Autodesk Inventor part; units mm, degrees
ref_plane "YZ Plane" through (0, 0, 0) normal (1, 0, 0) x (0, 1, 0)
ref_plane "XZ Plane" through (0, 0, 0) normal (0, 1, 0) x (-1, 0, 0)
ref_plane "XY Plane" through (0, 0, 0) normal (0, 0, 1) x (1, 0, 0)
sketch "Skizze1" plane through (0, 0, 0) normal (0, 0, 1) x (1, 0, 0)
  line L0 (0, 0) -> (84, 0)
  line L1 (84, 0) -> (84, 48)
  line L2 (84, 48) -> (0, 48)
  line L3 (0, 48) -> (0, 0)
  dimension "d0" = 48
  dimension "d1" = 84
extrude "Extrusion1" add sketch "Skizze1" along normal blind 4
sketch "Skizze2" plane through (0, 0, 4) normal (0, 0, 1) x (1, 0, 0)
  line L0 (0, 48) -> (0, 0)
  line L1 (0, 0) -> (84, 0)
  line L2 (84, 0) -> (84, 48)
  point P0 (4, 12)
  point P1 (4, 42)
  point P2 (80, 42)
  point P3 (80, 12)
  dimension "d4" = 4
  dimension "d5" = 30
  dimension "d6" = 12
  dimension "d7" = 4
hole "Bohrung1" at (4, 12, 4) at (4, 42, 4) at (80, 42, 4) at (80, 12, 4) direction (0, 0, -1) diameter 4 depth 4
sketch "Skizze3" plane through (0, 0, 4) normal (0, 0, 1) x (1, 0, 0)
  line L0 (0, 0) -> (84, 0)
  line L1 (0, 48) -> (0, 0)
  point P0 (24, 4)
  point P1 (60, 4)
  dimension "d15" = 4
  dimension "d16" = 24
  dimension "d17" = 36
hole "Bohrung2" at (24, 4, 4) at (60, 4, 4) direction (0, 0, -1) diameter 4 depth 4
properties part number "1012"
The model under review builds one solid part; all positions refer to its coordinate system, in mm. Round coordinates to 2 decimals unless told otherwise and drop trailing zeros. Order: outer loops, then holes, each group sorted by start corner. A loop starts at its lowest first (then second) coordinate and runs counter-clockwise, first axis right, second up. Notation, with made-up numbers: (19, -12.5) -> (64, -12.5) arc R8 ccw to (64, -7.5) -> close; hole circle Ø1 at (-28, 1). An arc over 180 degrees is marked (long way). Use a Markdown table: item, result.
Q1. We need section C-C on z = 2.8. Write out the cut boundary in (x, y), then the cut area to 3 significant figures.
Values:
| item | result |
|---|---|
| outline | (0, 0) -> (84, 0) -> (84, 48) -> (0, 48) -> close; hole circle Ø4 at (4, 12); hole circle Ø4 at (4, 42); hole circle Ø4 at (24, 4); hole circle Ø4 at (60, 4); hole circle Ø4 at (80, 12); hole circle Ø4 at (80, 42) |
| area | 3,960 mm^2 |
Q2. Clearance check with a flat-ended pin moving along its axis: P1, Ø3.5, axis at x = 4, y = 42, coming from the -Z side. State where the tip first meets the part, or that it passes through.
Values:
| item | result |
|---|---|
| P1 | passes through |
Q3. We need section B-B on y = 12. Write out the cut boundary in (x, z).
Values:
| item | result |
|---|---|
| outline | (0, 0) -> (2, 0) -> (2, 4) -> (0, 4) -> close; (6, 0) -> (78, 0) -> (78, 4) -> (6, 4) -> close; (82, 0) -> (84, 0) -> (84, 4) -> (82, 4) -> close |
Q4. For line 1 (Y direction, x = 80, z = 1.8); line 2 (X direction, y = 42, z = 1.8); line 3 (X direction, y = 4, z = 0.9), list the stretches that pass through material, from the lowest coordinate up.
Values:
| item | result |
|---|---|
| line 1 | y = 0 to 10, 14 to 40, 44 to 48 |
| line 2 | x = 0 to 2, 6 to 78, 82 to 84 |
| line 3 | x = 0 to 22, 26 to 58, 62 to 84 |
Q5. We need section D-D on x = 24. Write out the cut boundary in (y, z).
Values:
| item | result |
|---|---|
| outline | (0, 0) -> (2, 0) -> (2, 4) -> (0, 4) -> close; (6, 0) -> (48, 0) -> (48, 4) -> (6, 4) -> close |
Q6. We need section A-A on x = 4. Write out the cut boundary in (y, z).
Values:
| item | result |
|---|---|
| outline | (0, 0) -> (10, 0) -> (10, 4) -> (0, 4) -> close; (14, 0) -> (40, 0) -> (40, 4) -> (14, 4) -> close; (44, 0) -> (48, 0) -> (48, 4) -> (44, 4) -> close |
Q7. Mouldability with a two-part tool opening along Y and no side actions: class faces 1 (the flat face through (41, 24, 0)), 2 (the cylindrical face through (22.648, 5.474, 1.972)), 3 (the flat face through (43, 48, 2)) as +Y half, -Y half, draft (parallel to the pull), parting line (faces both ways), or undercut.
Values:
| item | result |
|---|---|
| face 1 | draft |
| face 2 | undercut |
| face 3 | +Y half |
